Read the model definition and answer for the solid it produces. Units are mm, in the model's axes. A direction names the side the tool comes from. Round coordinates to 2 decimals unless told otherwise and drop trailing zeros. Order: outer loops, then holes, each group sorted by start corner. A loop starts at its lowest first (then second) coordinate and runs counter-clockwise, first axis right, second up.
from build123d import *

# Parameters (mm, degrees)
BASPROSKE_W         = 4
BASPROSKE_H         = 10
TOOTHCUT_DEPTH      = 15.696938457
TEETHCUTS_COUNT     = 18
TEETHCUTS_ANGLE     = 340
BORSKE_R            = 2
BORE_DEPTH          = 50.0000508
SKETCH_1_R          = 9
EXTRUDE_1_DEPTH     = 4
SKETCH_2_R          = 2
CUT_EXTRUDE_1_DEPTH = 17.179282483
CUT_EXTRUDE_2_DEPTH = 3
SKETCH_6_R          = 2.9
EXTRUDE_2_DEPTH     = 5
SKETCH_7_R          = 2.1
CUT_EXTRUDE_3_DEPTH = 20.151218803


with BuildPart() as part:
    # BasProSke → Base-Revolve (revolve)
    with BuildSketch(Plane(origin=(0, 0, 0), x_dir=(1, 0, 0), z_dir=(0, 1, 0)), mode=Mode.PRIVATE) as base_revolve_sk:
        with Locations((2, 5)):
            Rectangle(BASPROSKE_W, BASPROSKE_H)
    revolve(base_revolve_sk.sketch.rotate(Axis((-10, 0, 0), (1, 0, 0)), 180), axis=Axis((-10, 0, 0), (1, 0, 0)))

    # TooCutSke → ToothCut (cut, through all)
    with BuildSketch(Plane(origin=(0, 0, 0), x_dir=(0, 0, -1), z_dir=(1, 0, 0))):
        with BuildLine():
            ThreePointArc((0.510641536, 7.732156635), (0, 7.749), (-0.510641536, 7.732156635))
            ThreePointArc((-0.510641536, 7.732156635), (-0.82619259, 8.907320741), (-1.515208602, 9.910236529))
            ThreePointArc((-1.515208602, 9.910236529), (0, 10.0254), (1.515208602, 9.910236529))
            ThreePointArc((1.515208602, 9.910236529), (0.82619259, 8.907320741), (0.510641536, 7.732156635))
        make_face()
    toothcut = extrude(amount=TOOTHCUT_DEPTH, mode=Mode.SUBTRACT)

    # TeethCuts: ToothCut ×18 about axis
    teethcuts_axis = Axis((-10, 0, 0), (1, 0, 0))
    for i in range(1, TEETHCUTS_COUNT):
        add(toothcut.rotate(teethcuts_axis, i * TEETHCUTS_ANGLE / (TEETHCUTS_COUNT - 1)), mode=Mode.SUBTRACT)

    # BorSke → Bore (cut, symmetric)
    with BuildSketch(Plane(origin=(0, 0, 0), x_dir=(0, 0, -1), z_dir=(1, 0, 0))):
        with Locations(Location((0, 0, 0), (0, 0, 180))):
            Circle(BORSKE_R)
    extrude(amount=BORE_DEPTH, both=True, mode=Mode.SUBTRACT)

    # 草图1 → 凸台-拉伸1 (add)
    with BuildSketch(Plane.ZY):
        with Locations(Location((0, 0, 0), (0, 0, 184.575164613))):
            Circle(SKETCH_1_R)
    extrude(amount=EXTRUDE_1_DEPTH)

    # 草图2 → 切除-拉伸1 (cut, through all)
    with BuildSketch(Plane.ZY.offset(4)):
        Circle(SKETCH_2_R)
    extrude(amount=-CUT_EXTRUDE_1_DEPTH, mode=Mode.SUBTRACT)

    # 草图3 → 切除-拉伸2 (cut)
    with BuildSketch(Plane.ZY.offset(4)):
        Polygon((6.2, 3.579571669), (0, 7.159143338), (-6.2, 3.579571669), (-6.2, -3.579571669), (0, -7.159143338), (6.2, -3.579571669), align=None)
    extrude(amount=-CUT_EXTRUDE_2_DEPTH, mode=Mode.SUBTRACT)

    # 草图6 → 凸台-拉伸2 (add)
    with BuildSketch(Plane(origin=(4, 0, 0), x_dir=(0, 0, -1), z_dir=(1, 0, 0))):
        with Locations(Location((0, 0, 0), (0, 0, 180))):
            Circle(SKETCH_6_R)
    extrude(amount=EXTRUDE_2_DEPTH)

    # 草图7 → 切除-拉伸3 (cut, through all)
    with BuildSketch(Plane(origin=(9, 0, 0), x_dir=(0, 0, -1), z_dir=(1, 0, 0))):
        Circle(SKETCH_7_R)
    extrude(amount=-CUT_EXTRUDE_3_DEPTH, mode=Mode.SUBTRACT)


solid = part.part
Q1. A cutting plane is placed at A-A, the plane x = -2.5. Give the vertices of the cut face in (y, z).
Outcome:
outline: circle Ø18 at (0, 0); hole (-7.16, 0) - (-3.58, -6.2) - (3.58, -6.2) - (7.16, 0) - (3.58, 6.2) - (-3.58, 6.2) - close
Q2. Flat-ended cylindrical pins translate along their axes: pin 1 (4 mm diameter, centred on y = 5.5, z = 6, fed in from +X); pin 2 (4 mm diameter, centred on x = 0, y = 7.5, fed in from -Z); pin 3 (3 mm diameter, centred on x = 0.5, y = 0.5, fed in from -Z); pin 4 (1 mm diameter, centred on y = 8.5, z = 0, fed in from +X). Find the tip coordinate at first contact, or state that the pin passes through.
Outcome:
pin 1: stops at x = 4
pin 2: stops at z = -7.82
pin 3: stops at z = -10
pin 4: stops at x = 0
Q3. Straight lines are drawn through the part: probe 1 along Y at (x, z) = (5.5, 0); probe 2 along X at (y, z) = (2.5, -4.5); probe 3 along X at (y, z) = (-5, 6.25). For each, find the intervals that lie inside material, in ascending order.
Outcome:
probe 1: y = -2.9 to -2.1, 2.1 to 2.9
probe 2: x = -1 to 4
probe 3: x = -4 to 4
Q4. A cutting plane is placed at B-B, the plane z = 4.25. Give the vertices of the cut face in (x, y).
Outcome:
outline: (-4, -7.93) - (0, -7.93) - (0, -8.46) - (4, -8.46) - (4, 8.46) - (0, 8.46) - (0, 7.93) - (-4, 7.93) - (-4, 4.71) - (-1, 4.71) - (-1, -4.71) - (-4, -4.71) - close
Q5. For faces 1 (the face through (0, 8, 0)), 2 (the face through (-2.521, -5.394, 3.057)), 3 (the face through (1.97, 2.36, 8.63)), 4 (the face through (1.972, -8.878, -0.813)), 5 (the face through (1.972, -3.735, -8.095)), determine the directions among +Z, -Z, +X, -X, +Y, -Y from which every point of the face is accessible in a straight line to the end or side of a thin tool.
Outcome:
face 1: +X, +Y
face 2: -X
face 3: +Z, +X
face 4: +X, -Y
face 5: +X
Q6. A cutting plane is placed at C-C, the plane x = 5.25. Give the vertices of the cut face in (y, z), plus the area to 3 significant figures.
Outcome:
outline: circle Ø5.8 at (0, 0); hole circle Ø4.2 at (0, 0)
area: 12.6 mm2
